Verification items for the finished model (mm, model axes). A direction names the side the tool comes from. Give positions to 0.01 mm unless a question says otherwise; leave off trailing zeros. Loops run counter-clockwise (first coordinate to the right, second up) from the corner with the lowest first, then second, coordinate; pieces in that order, holes last. Notation, with made-up numbers: (44.5, 21.5) - (90.5, 21.5) arc R20 ccw to (90.5, 47.5) - close; hole circle Ø1 at (34, 83.5). An arc over 180 degrees is marked (long way). One line per question, with ' | ' between items. Start each with the question number.
1. Mould release check, pull along X, two halves, no side actions. Record for faces 1 (the face through (0, 3, 1.2)), 2 (the face through (1.5, 0.07, 0.25)): +X half, -X half, draft (parallel to the pull), parting line (faces both ways), or undercut.
2. Tool access check on faces 3 (the face through (1.2, -1.2, 0)), 4 (the face through (0, -3, 1.2)), 5 (the face through (0, 0, 0.5)). Record the directions out of +Z, -Z, +X, -X, +Y, -Y that give a thin tool (end or side, any length) a straight path to the whole face; none if there is none.
3. Section check A-A, the plane x = 0. Enter the section's corners in (y, z), then the cut area to 3 significant figures.
4. Thickness scan on line 1 along Y through (x, z) = (0, 0.2); line 2 along Y through (x, z) = (-3, 1.9); line 3 along Z through (x, y) = (-4.75, -1.5). Record the ranges inside material, lowest first. Write a range as from..to.
5. Section check C-C, the plane z = 0.8. Enter the section's corners in (x, y), then the cut area to 3 significant figures.
6. Section check D-D, the plane x = 3.5. Enter the section's corners in (y, z), then the cut area to 3 significant figures.
7. Section check B-B, the plane y = 0. Enter the section's corners in (x, z), then the cut area to 3 significant figures.
8. Depth check by flat-ended pin: pin 1 Ø6 at (x, y) = (2, -3.5) entering from +Z; pin 2 Ø2.5 at (x, y) = (0, 0) entering from -Z; pin 3 Ø1.4 at (x, y) = (-1.5, 3.5) entering from +Z; pin 4 Ø5 at (x, y) = (4, -3.5) entering from +Z. Enter the tip coordinate at first touch or a pass-through.
from build123d import *

# Parameters (mm, degrees)
SKETCH1_R           = 5.9
BOSS_EXTRUDE1_DEPTH = 1.2
BOSS_EXTRUDE2_DEPTH = 0.8
CHAMFER1_SIZE       = 0.4
SKETCH3_R           = 1.5
CUT_EXTRUDE1_DEPTH  = 0.5


with BuildPart() as part:
    # Sketch1 → Boss-Extrude1 (new body)
    with BuildSketch(Plane.XY):
        Circle(SKETCH1_R)
    extrude(amount=BOSS_EXTRUDE1_DEPTH)

    # Sketch2 → Boss-Extrude2 (add)
    with BuildSketch(Plane.XY.offset(1.2)):
        with BuildLine():
            Line((-5.852136362, -0.75), (5.852136362, -0.75))
            ThreePointArc((5.852136362, -0.75), (5.9, 0), (5.852136362, 0.75))
            Line((5.852136362, 0.75), (-5.852136362, 0.75))
            ThreePointArc((-5.852136362, 0.75), (-5.9, 0), (-5.852136362, -0.75))
        make_face()
    extrude(amount=BOSS_EXTRUDE2_DEPTH)

    # Chamfer1
    # the kernel refuses this chamfer: 0.4 mm, written as the material it adds along each edge
    with BuildSketch(Plane(origin=(6.880809557, 0.75, 1.2), x_dir=(0, 0.9996219169112968, -0.02749587661058628), z_dir=(-1, 0, 0))) as chamfer1_piece_1_section:
        Polygon((CHAMFER1_SIZE * 0.999621916911, -CHAMFER1_SIZE * 0.0274958766106), (-CHAMFER1_SIZE * 0.0274958766106, -CHAMFER1_SIZE * 0.999621916911), (0, 0), align=None)
    chamfer1_piece_1 = extrude(amount=13.761619114, mode=Mode.PRIVATE)
    chamfer1_piece_1 = chamfer1_piece_1 & Plane(origin=(0, 0, 1.33206261), x_dir=(1, 0, 0), z_dir=(0, 0, -1)) * Cylinder(5.9, 30, mode=Mode.PRIVATE)
    add(chamfer1_piece_1)
    with BuildSketch(Plane(origin=(-6.880809557, -0.75, 1.2), x_dir=(0, -0.9996219169112968, -0.027495876610586285), z_dir=(1, 0, 0))) as chamfer1_piece_2_section:
        Polygon((CHAMFER1_SIZE * 0.999621916911, -CHAMFER1_SIZE * 0.0274958766106), (-CHAMFER1_SIZE * 0.0274958766106, -CHAMFER1_SIZE * 0.999621916911), (0, 0), align=None)
    chamfer1_piece_2 = extrude(amount=13.761619114, mode=Mode.PRIVATE)
    chamfer1_piece_2 = chamfer1_piece_2 & Plane(origin=(0, 0, 1.33206261), x_dir=(1, 0, 0), z_dir=(0, 0, -1)) * Cylinder(5.9, 30, mode=Mode.PRIVATE)
    add(chamfer1_piece_2)

    # Sketch3 → Cut-Extrude1 (cut)
    with BuildSketch(Plane(origin=(0, 0, 0), x_dir=(-1, 0, 0), z_dir=(0, 0, -1))):
        Circle(SKETCH3_R)
    extrude(amount=-CUT_EXTRUDE1_DEPTH, mode=Mode.SUBTRACT)


solid = part.part
Results list:
1) face 1: draft | face 2: undercut
2) face 3: -Z, +X, -X, +Y, -Y | face 4: +Z, +X, -X, -Y | face 5: -Z
3) outline: (-5.9, 0) - (-1.5, 0) - (-1.5, 0.5) - (1.5, 0.5) - (1.5, 0) - (5.9, 0) - (5.9, 1.2) - (1.15, 1.2) - (0.75, 1.6) - (0.75, 2) - (-0.75, 2) - (-0.75, 1.6) - (-1.15, 1.2) - (-5.9, 1.2) - close | area: 14.0 mm²
4) line 1: -5.9..-1.5, 1.5..5.9 | line 2: -0.75..0.75 | line 3: 0..1.2
5) outline: circle Ø11.8 at (0, 0) | area: 109 mm²
6) outline: (-4.75, 0) - (4.75, 0) - (4.75, 1.2) - (1.15, 1.2) - (0.75, 1.6) - (0.75, 2) - (-0.75, 2) - (-0.75, 1.6) - (-1.15, 1.2) - (-4.75, 1.2) - close | area: 12.8 mm²
7) outline: (-5.9, 0) - (-1.5, 0) - (-1.5, 0.5) - (1.5, 0.5) - (1.5, 0) - (5.9, 0) - (5.9, 2) - (-5.9, 2) - close | area: 22.1 mm²
8) pin 1: z = 2 | pin 2: z = 0.5 | pin 3: z = 1.2 | pin 4: z = 1.35
